Could you check a few things on this model? Use its own coordinates, in mm. A direction names the side the tool comes from. Give positions to 0.01 mm unless a question says otherwise; leave off trailing zeros. Loops run counter-clockwise (first coordinate to the right, second up) from the corner with the lowest first, then second, coordinate; pieces in that order, holes last. Notation, with made-up numbers: M 3.25,36 L 24.25,36 A16 cw 24.25,64 Z; hole C 57.5,52 d4. An arc over 180 degrees is marked long. Use CSV: the item, a comma, the result in double quotes.
```python
from build123d import *

# Parameters (mm, degrees)
SKETCH1_R               = 0.6
CUT_EXTRUDE1_DEPTH      = 2
CIRPATTERN1_COUNT       = 4
ESQUISSE2_R             = 0.934495928
ESQUISSE2_R_2           = 0.971023647
ESQUISSE2_R_3           = 0.919680735
ESQUISSE2_R_4           = 0.940854572
ENL_V_MAT_EXTRU_1_DEPTH = 15.361406616


with BuildPart() as part:
    # Esquisse1 → Révolution1 (revolve)
    with BuildSketch(Plane.XY, mode=Mode.PRIVATE) as r_volution1_sk:
        Polygon((2.75, 0), (2.75, 3), (1.5, 3), (1.5, 4), (3, 4), (3, 5), (3.75, 5), (3.75, 4.5), (10, 4.5), (10, 2.5), (4.5, 2.5), (4.5, 0), align=None)
    revolve(r_volution1_sk.sketch.rotate(Axis((0, 0, 0), (0, 1, 0)), 90), axis=Axis((0, 0, 0), (0, 1, 0)))

    # Sketch1 → Cut-Extrude1 (cut)
    with BuildSketch(Plane(origin=(0, 4.5, 0), x_dir=(1, 0, 0), z_dir=(0, 1, 0))):
        with Locations(Location((0, 7.5, 0), (0, 0, 270))):
            Circle(SKETCH1_R)
        with Locations(Location((3, 7.5, 0), (0, 0, 270))):
            Circle(SKETCH1_R)
        with Locations(Location((-3, 7.5, 0), (0, 0, 90))):
            Circle(SKETCH1_R)
    cut_extrude1 = extrude(amount=-CUT_EXTRUDE1_DEPTH, mode=Mode.SUBTRACT)

    # CirPattern1: Cut-Extrude1 ×4 about axis
    cirpattern1_axis = Axis((0, 0, 0), (0, 1, 0))
    for i in range(1, CIRPATTERN1_COUNT):
        add(cut_extrude1.rotate(cirpattern1_axis, i * 360 / CIRPATTERN1_COUNT), mode=Mode.SUBTRACT)

    # Esquisse2 → Enlèv. mat.-Extru.1 (cut, through all)
    with BuildSketch(Plane.XZ.offset(-2.5)):
        with Locations(Location((0, -7.5, 0), (0, 0, 270))):
            Circle(ESQUISSE2_R)
        with Locations(Location((-7.5, 0, 0), (0, 0, 270))):
            Circle(ESQUISSE2_R_2)
        with Locations(Location((0, 7.5, 0), (0, 0, 270))):
            Circle(ESQUISSE2_R_3)
        with Locations(Location((7.5, 0, 0), (0, 0, 270))):
            Circle(ESQUISSE2_R_4)
    extrude(amount=-ENL_V_MAT_EXTRU_1_DEPTH, mode=Mode.SUBTRACT)


solid = part.part
```
1. Please list where these lines run through material, in increasing order: line 1 (X direction, y = 3.3, z = 0); line 2 (Z direction, x = -7.75, y = 3.35); line 3 (X direction, y = 1.25, z = 0).
Outcome:
line 1,"-10 to -8.47, -6.53 to -1.5, 1.5 to 6.56, 8.44 to 10"
line 2,"-6.32 to -3.55, -2.45 to -0.94, 0.94 to 2.45, 3.55 to 6.32"
line 3,"-4.5 to -2.75, 2.75 to 4.5"
2. I'm going to push flat-ended pins straight in: pin 1 Ø1.9 at (x, z) = (-7.5, 3) entering from +Y; pin 2 Ø1.6 at (x, z) = (-3, -7.5) entering from -Y; pin 3 Ø4.5 at (x, z) = (0, 0) entering from -Y. Where does each tip first touch, or does it pass through?
Outcome:
pin 1,"y = 4.5"
pin 2,"y = 2.5"
pin 3,"y = 3"
3. I want a section at A-A, the plane z = 0. Give the number of separate pieces and of enclosed holes in the cut face, then the cut area to 3 significant figures.
Outcome:
separate pieces,"4"
enclosed holes,"0"
area,"33.1 mm2"
4. If we mould it in two halves opening along X, with no side actions, what happens to faces 4 (the face through (0, 3, 10)), 5 (the face through (-3, 5, 1)), 6 (the face through (-3, 3.5, 8.1))? For each: +X half, -X half, draft (parallel to the pull), parting line (faces both ways), or undercut.
Outcome:
face 4,"parting line"
face 5,"draft"
face 6,"undercut"
5. I want a section at C-C, the plane z = 3.25. List the corners of the cut face in (x, y) for me.
Outcome:
outline,"M -9.46,2.5 L -8.05,2.5 L -8.05,4.5 L -9.46,4.5 Z; M -6.95,2.5 L -3.11,2.5 L -3.11,0 L 3.11,0 L 3.11,2.5 L 6.95,2.5 L 6.95,4.5 L 1.87,4.5 L 1.87,5 L -1.87,5 L -1.87,4.5 L -6.95,4.5 Z; M 8.05,2.5 L 9.46,2.5 L 9.46,4.5 L 8.05,4.5 Z"
6. Which directions (+Z, -Z, +X, -X, +Y, -Y) give clear straight access to the entire face, cutting with the end or side of a thin tool? Please do faces 1 (the face through (-3.16, 4.75, -2.02)), 2 (the face through (6.665, 3.486, -0.434)), 3 (the face through (-3.04, 1.23, 3.32)).
Outcome:
face 1,"+Y"
face 2,"+Y, -Y"
face 3,"-Y"
